Autodesk Inventor part; units mm, degrees
ref_plane "YZ Plane" through (0, 0, 0) normal (1, 0, 0) x (0, 1, 0)
ref_plane "XZ Plane" through (0, 0, 0) normal (0, 1, 0) x (-1, 0, 0)
ref_plane "XY Plane" through (0, 0, 0) normal (0, 0, 1) x (1, 0, 0)
sketch "スケッチ1" plane through (0, 0, 0) normal (0, 0, 1) x (1, 0, 0)
  circle A0 centre (0, 0) radius 10.5 construction
  line L0 (0, 10.5) -> (-200, 10.5) construction
  line L1 (-200, 10.5) -> (-200, -10.5) construction
  line L2 (-200, -10.5) -> (0, -10.5) construction
  circle A1 centre (-195, 0) radius 1.55 construction
  line L3 (-185, 2.5) -> (-70, 2.5) construction
  line L4 (-70, 2.5) -> (-70, -2.5) construction
  line L5 (-70, -2.5) -> (-185, -2.5) construction
  line L6 (-185, -2.5) -> (-185, 2.5) construction
  line L7 (-127.5, 2.5) -> (-127.5, -2.5) construction
  circle A2 centre (-60, 0) radius 1.55 construction
  line L8 (-12, 21.3027) -> (-12, -27.3903) construction
  line L9 (-69.95, 2.55) -> (-185.05, 2.55) construction
  line L10 (-185.05, 2.55) -> (-185.05, -2.55) construction
  line L11 (-185.05, -2.55) -> (-69.95, -2.55) construction
  line L12 (-69.95, -2.55) -> (-69.95, 2.55) construction
  circle A3 centre (-184, 2.55) radius 1.05 construction
  line L13 (-185, 0) -> (-127.5, 0) construction
  line L14 (-185.05, 2.55) -> (-185.05, -2.55) construction
  arc A4 (-182.95, 2.55) -> (-185.05, 2.55) centre (-184, 2.55) ccw construction
  line L15 (-182.95, 2.55) -> (-72.05, 2.55) construction
  arc A5 (-69.95, 2.55) -> (-72.05, 2.55) centre (-71, 2.55) ccw construction
  line L16 (-69.95, 2.55) -> (-69.95, -2.55) construction
  arc A6 (-185.05, -2.55) -> (-182.95, -2.55) centre (-184, -2.55) ccw construction
  line L17 (-182.95, -2.55) -> (-72.05, -2.55) construction
  arc A7 (-72.05, -2.55) -> (-69.95, -2.55) centre (-71, -2.55) ccw construction
  circle A8 centre (0, 8.5) radius 1.35
  circle A9 centre (0, 0) radius 5.05
  circle A10 centre (-8.5, 0) radius 1.35
  circle A11 centre (0, -8.5) radius 1.35
  circle A12 centre (8.5, 0) radius 1.35
  line L18 (-200, 4.8006) -> (-200, -4.8006) construction
  line L19 (-200, 4.8006) -> (-60, 10.5) construction
  line L20 (-60, 10.5) -> (0, 10.5) construction
  line L21 (-200, -4.8006) -> (-60, -10.5) construction
  line L22 (-60, -10.5) -> (0, -10.5) construction
  arc A13 (0, -10.5) -> (0, 10.5) centre (0, 0) ccw construction
  circle A14 centre (-195, 0) radius 5 construction
  circle A15 centre (-59, 0) radius 1.55
  circle A16 centre (-84, 0) radius 1.55
  line L23 (-55, -2.5) -> (-88, -2.5) construction
  line L24 (-88, -2.5) -> (-88, 2.5) construction
  line L25 (-88, 2.5) -> (-55, 2.5) construction
  line L26 (-55, 2.5) -> (-55, -2.5) construction
  line L27 (-65, -2.5) -> (-78, -2.5) construction
  line L28 (-78, -2.5) -> (-78, 2.5) construction
  line L29 (-78, 2.5) -> (-65, 2.5) construction
  line L30 (-65, 2.5) -> (-65, -2.5) construction
  line L31 (-64.95, -2.55) -> (-78.05, -2.55)
  line L32 (-78.05, -2.55) -> (-78.05, 2.55)
  line L33 (-78.05, 2.55) -> (-64.95, 2.55)
  line L34 (-64.95, 2.55) -> (-64.95, -2.55)
  circle A17 centre (-66, -2.55) radius 1.05
  circle A18 centre (-66, 2.55) radius 1.05
  circle A19 centre (-77, -2.55) radius 1.05
  circle A20 centre (-77, 2.55) radius 1.05
  line L35 (-88, 2.5) -> (-88, -2.5)
  line L36 (-88, -2.5) -> (-54.4113, -10.5)
  line L37 (-88, 2.5) -> (-54.4113, 10.5)
  arc A21 (0, -10.5) -> (0, 10.5) centre (0, 0) ccw
  line L38 (-54.4113, 10.5) -> (0, 10.5)
  line L39 (0, -10.5) -> (-54.4113, -10.5)
  circle A22 centre (-77, 2.55) radius 2.5 construction
  circle A23 centre (0, 0) radius 16 construction
  circle A24 centre (0, 0) radius 21 construction
  line L40 (-21, 19.3585) -> (-21, -28.09) construction
  point P0 (-200, 0)
  point P1 (-55, 0)
  dimension "d9" = 2.1
  dimension "d29" = 2.1
  dimension "d0" = 200
  dimension "d1" = 3.1
  dimension "d2" = 21
  dimension "d3" = 10
  dimension "d4" = 5
  dimension "d5" = 12
  dimension "d6" = 135
  dimension "d7" = 5
  dimension "d8" = 0.05
  dimension "d10" = 2.7
  dimension "d11" = 8.5
  dimension "d12" = 10.1
  dimension "d15" = 360
  dimension "d20" = 3.1
  dimension "d21" = 5
  dimension "d22" = 4
  dimension "d23" = 5
  dimension "d24" = 25
  dimension "d26" = 10
  dimension "d27" = 4
  dimension "d28" = 10
  dimension "d30" = 0.05
  dimension "d32" = 5
  dimension "d33" = 32
  dimension "d34" = 5
extrude "押し出し1" add sketch "スケッチ1" along normal blind 2
fillet "フィレット2" radius 2 2 edges at (-88, 2.5, 1) (-88, -2.5, 1)
equation "\"d2\" = d2_1"
equation "\"d3\" = d3_1"
equation "\"d4\" = d4_1"
equation "\"d6\" = d6_1"
equation "\"d21\" = d4"
equation "\"d27\" = d22"
equation "\"d28\" = d26"
properties part number "ForeArm_inside_frame" material "GFRP"
Design review of the part built by this model. Coordinates are the model's own, in mm. A direction names the side the tool comes from. Round coordinates to 2 decimals unless told otherwise and drop trailing zeros. Write each loop counter-clockwise with the first axis right and the second up, starting at its lowest first coordinate (ties: lowest second). Pieces come first, ordered by that corner, then holes.
Item 1: The part is to be moulded in two halves that separate along X. For faces 1 (the cylindrical face through (-66, -3.6, 1)), 2 (the flat face through (-28, 0, 2)), 3 (the flat face through (-78.05, 0, 1)), 4 (the flat face through (-88, 0, 1)), say which applies: +X half, -X half, draft (parallel to the pull), parting line (faces both ways), or undercut.
Item 2: We need section C-C on z = 0.95. State how many separate pieces and enclosed holes the cut face has, and give its area (3 significant figures).
Item 3: For faces 5 (the cylindrical face through (10.5, 0.2, 1)), 6 (the cylindrical face through (-66, 3.6, 1)), list the 3-axis set-ups (+Z, -Z, +X, -X, +Y, -Y) from which the entire face can be reached by the end or side of a thin tool; tool diameter is ignored.
Item 4: We need section B-B on y = 0. Write out the cut boundary in (x, z), and give its area (3 significant figures).
Item 5: We need section D-D on y = -8.5. Write out the cut boundary in (x, z).
Item 6: For probe 1 along Y at (x, z) = (0, 1.15); probe 2 along Y at (x, z) = (-8.5, 1); probe 3 along Y at (x, z) = (3, 0.4), list the stretches that pass through material, from the lowest coordinate up.
Item 7: Clearance check with flat-ended pins moving along their axes: pin 1 Ø2.5 at (x, y) = (0, -8.5) entering from -Z; pin 2 Ø1 at (y, z) = (-1, 1.5) entering from +X; pin 3 Ø0.6 at (x, z) = (-72, 1) entering from -Y. State where each tip first meets the part, or that it passes through.
Item 8: We need section A-A on x = -8.5. Write out the cut boundary in (y, z), and give its area (3 significant figures).
Returned:
1. face 1: undercut
1. face 2: draft
1. face 3: undercut
1. face 4: -X half
2. separate pieces: 1
2. enclosed holes: 8
2. area: 1,560 mm2
3. face 5: +Z, -Z, +X
3. face 6: +Z, -Z
4. outline: (-88, 0) - (-85.55, 0) - (-85.55, 2) - (-88, 2) - close; (-82.45, 0) - (-78.05, 0) - (-78.05, 2) - (-82.45, 2) - close; (-64.95, 0) - (-60.55, 0) - (-60.55, 2) - (-64.95, 2) - close; (-57.45, 0) - (-9.85, 0) - (-9.85, 2) - (-57.45, 2) - close; (-7.15, 0) - (-5.05, 0) - (-5.05, 2) - (-7.15, 2) - close; (5.05, 0) - (7.15, 0) - (7.15, 2) - (5.05, 2) - close; (9.85, 0) - (10.5, 0) - (10.5, 2) - (9.85, 2) - close
4. area: 127 mm2
5. outline: (-62.81, 0) - (-1.35, 0) - (-1.35, 2) - (-62.81, 2) - close; (1.35, 0) - (6.16, 0) - (6.16, 2) - (1.35, 2) - close
6. probe 1: y = -10.5 to -9.85, -7.15 to -5.05, 5.05 to 7.15, 9.85 to 10.5
6. probe 2: y = -10.5 to -1.35, 1.35 to 10.5
6. probe 3: y = -10.06 to -4.06, 4.06 to 10.06
7. pin 1: passes through
7. pin 2: stops at x = 10.49
7. pin 3: stops at y = -6.38
8. outline: (-10.5, 0) - (-1.35, 0) - (-1.35, 2) - (-10.5, 2) - close; (1.35, 0) - (10.5, 0) - (10.5, 2) - (1.35, 2) - close
8. area: 36.6 mm2
